Verification items for this drawing (mm, ordinates from the low corner). Round coordinates to 2 decimals unless told otherwise and drop trailing zeros. Order: outer loops, then holes, each group sorted by start corner. A loop starts at its lowest first (then second) coordinate and runs counter-clockwise, first axis right, second up. Notation, with made-up numbers: (47, -15.75) -> (100, -15.75) arc R27 cw to (100, 11.25) -> close; hole circle Ø11 at (59.5, -27.5). An arc over 180 degrees is marked (long way). Answer in a Markdown table with one row per item. Add a question column.
1. Sectioned sample at B-B, the plane z = 1.6. Count the separate pieces of the cut face and the enclosed holes in it, then the cut area to 3 significant figures.
2. Sectioned sample at D-D, the plane x = 8.75. Record the boundary of the cut face in (y, z), then the cut area to 3 significant figures.
3. Sectioned sample at C-C, the plane x = 13.97. Record the boundary of the cut face in (y, z), then the cut area to 3 significant figures.
4. Material ranges on L1, parallel to Y at x = 11.43, z = 1.8; L2, parallel to Y at x = 6.5, z = 0.7, recorded low to high. Write a range as from..to.
5. Sectioned sample at A-A, the plane y = 1.27. Record the boundary of the cut face in (x, z), then the cut area to 3 significant figures.
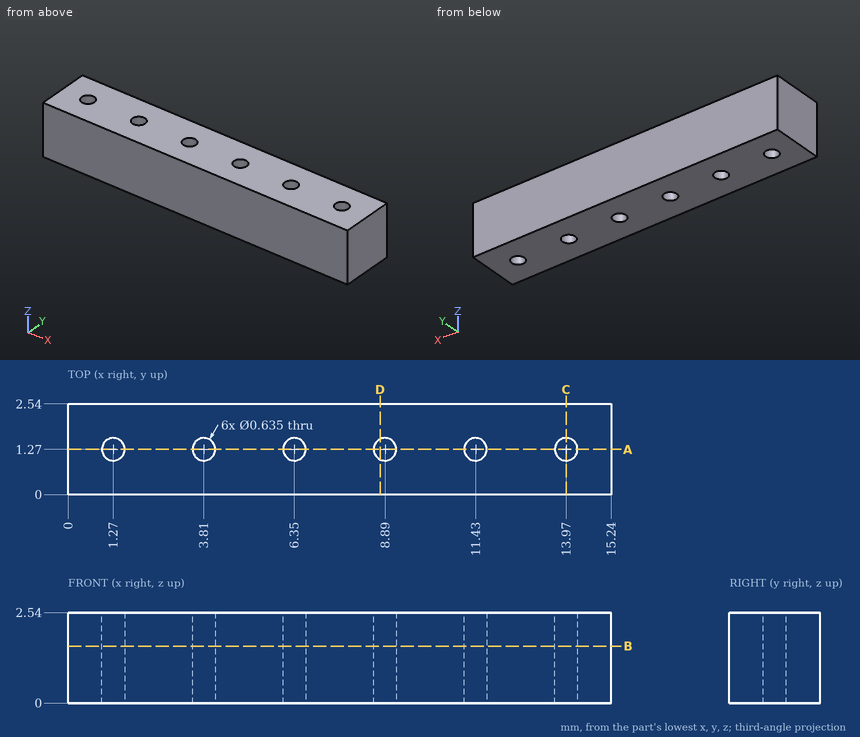
Answer key:
| question | item | result |
|---|---|---|
| 1 | separate pieces | 1 |
| 1 | enclosed holes | 6 |
| 1 | area | 36.8 mm² |
| 2 | outline | (0, 0) -> (0.99, 0) -> (0.99, 2.54) -> (0, 2.54) -> close; (1.55, 0) -> (2.54, 0) -> (2.54, 2.54) -> (1.55, 2.54) -> close |
| 2 | area | 5.00 mm² |
| 3 | outline | (0, 0) -> (0.95, 0) -> (0.95, 2.54) -> (0, 2.54) -> close; (1.59, 0) -> (2.54, 0) -> (2.54, 2.54) -> (1.59, 2.54) -> close |
| 3 | area | 4.84 mm² |
| 4 | L1 | y = 0..0.95, 1.59..2.54 |
| 4 | L2 | y = 0..0.99, 1.55..2.54 |
| 5 | outline | (0, 0) -> (0.95, 0) -> (0.95, 2.54) -> (0, 2.54) -> close; (1.59, 0) -> (3.49, 0) -> (3.49, 2.54) -> (1.59, 2.54) -> close; (4.13, 0) -> (6.03, 0) -> (6.03, 2.54) -> (4.13, 2.54) -> close; (6.67, 0) -> (8.57, 0) -> (8.57, 2.54) -> (6.67, 2.54) -> close; (9.21, 0) -> (11.11, 0) -> (11.11, 2.54) -> (9.21, 2.54) -> close; (11.75, 0) -> (13.65, 0) -> (13.65, 2.54) -> (11.75, 2.54) -> close; (14.29, 0) -> (15.24, 0) -> (15.24, 2.54) -> (14.29, 2.54) -> close |
| 5 | area | 29.0 mm² |
